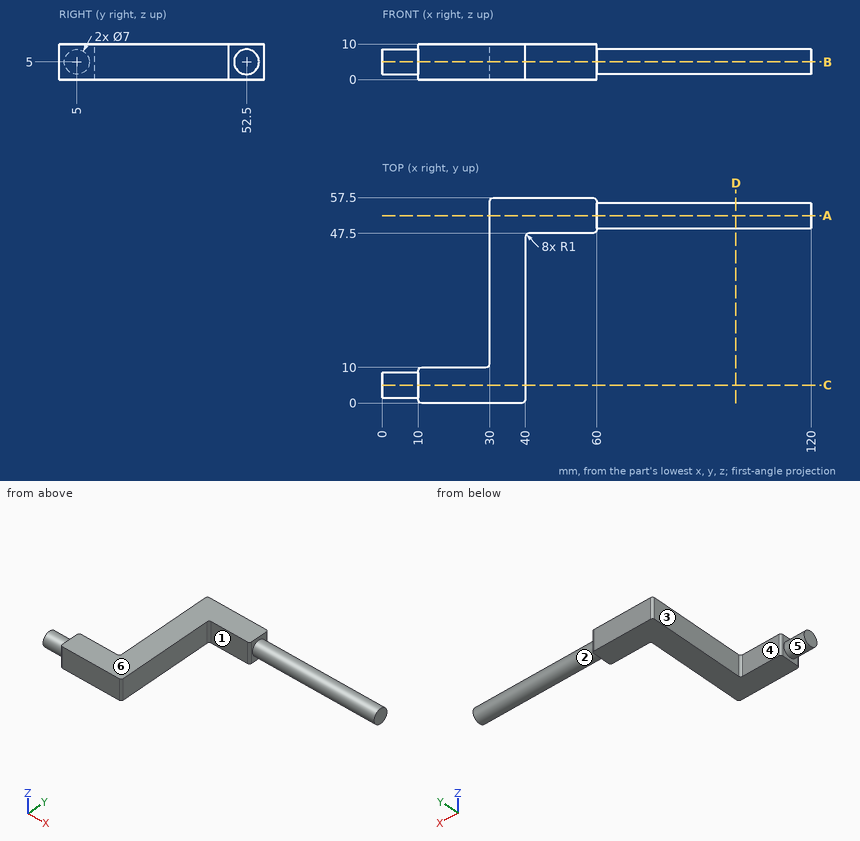
The drawing under review shows one solid part. Ordinate dimensions are in mm from its lowest x, y, z. A direction names the side the tool comes from. Round coordinates to 2 decimals unless told otherwise and drop trailing zeros. Write each loop counter-clockwise with the first axis right and the second up, starting at its lowest first coordinate (ties: lowest second). Pieces come first, ordered by that corner, then holes. Notation, with made-up numbers: (33, 69.5) - (85, 69.5) arc R17 cw to (85, 84.5) - close; hole circle Ø10 at (-38, 5.5). An arc over 180 degrees is marked (long way). Use one line per item in the form item = value.
Q1. Consider section D-D (x = 99). State the section outline as (y, z) points.
Answer key:
outline = circle Ø7 at (52.5, 5)
Q2. Consider section C-C (y = 5). State the section outline as (x, z) points.
Answer key:
outline = (0, 1.5) - (10, 1.5) - (10, 0) - (40, 0) - (40, 10) - (10, 10) - (10, 8.5) - (0, 8.5) - close
Q3. Insertion check: pin 1 Ø3 at (y, z) = (37, 1.5) entering from -X; pin 2 Ø4 at (x, z) = (22.5, 3.5) entering from +Y; pin 3 Ø1.5 at (y, z) = (12.5, 1.5) entering from +X. Each pin has a flat end and moves straight along its axis. Give the tip position at first contact, or say it passes through.
Answer key:
pin_1 = 30
pin_2 = 10
pin_3 = 40
Q4. Tool access review of the marked faces 1, 2 and 3: name each direction out of +Z, -Z, +X, -X, +Y, -Y from which nothing blocks a thin tool from reaching the whole face with its end or side.
Answer key:
face_1 = +Z, -Z, +X, -Y
face_2 = +X
face_3 = +Z, -Z, -X, +Y
Q5. Consider section A-A (y = 52.5). State the section outline as (x, z) points, and give its area (3 significant figures).
Answer key:
outline = (30, 0) - (60, 0) - (60, 1.5) - (120, 1.5) - (120, 8.5) - (60, 8.5) - (60, 10) - (30, 10) - close
area = 720 mm2
Q6. For line 1 (X direction, y = 16, z = 5.75); line 2 (X direction, y = 5, z = 4.5); line 3 (Y direction, x = 26, z = 7), list the stretches that pass through material, from the lowest coordinate up. Write a range as [from, to].
Answer key:
line_1 = [30, 40]
line_2 = [0, 40]
line_3 = [0, 10]
Q7. Consider section B-B (z = 5). State the section outline as (x, y) points.
Answer key:
outline = (0, 1.5) - (10, 1.5) - (10, 1) arc R1 ccw to (11, 0) - (39, 0) arc R1 ccw to (40, 1) - (40, 46.5) arc R1 cw to (41, 47.5) - (59, 47.5) arc R1 ccw to (60, 48.5) - (60, 49) - (120, 49) - (120, 56) - (60, 56) - (60, 56.5) arc R1 ccw to (59, 57.5) - (31, 57.5) arc R1 ccw to (30, 56.5) - (30, 11) arc R1 cw to (29, 10) - (11, 10) arc R1 ccw to (10, 9) - (10, 8.5) - (0, 8.5) - close
Q8. Draft analysis for pull direction Z (two halves, no side actions). For the marked faces 4, 5 and 6, state which applies: +Z half, -Z half, draft (parallel to the pull), parting line (faces both ways), or undercut.
Answer key:
face_4 = draft
face_5 = parting line
face_6 = +Z half
